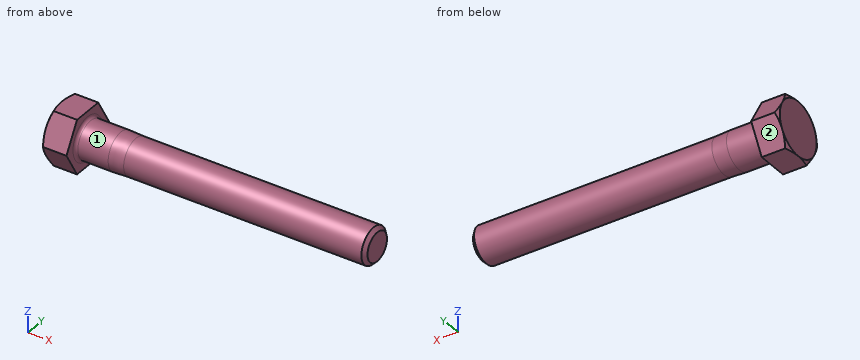
Autodesk Inventor part; units mm, degrees
ref_plane "Work Plane1" through (1.525, 0, 0) normal (0, 0, 1) x (1, 0, 0)
ref_plane "YZ Plane" through (0, 0, 0) normal (1, 0, 0) x (0, 1, 0)
ref_plane "XZ Plane" through (0, 0, 0) normal (0, 1, 0) x (-1, 0, 0)
sketch "Sketch1" plane through (0, 0, 0) normal (0, 0, 1) x (1, 0, 0)
  line L0 (0, 7.1374) -> (0, 4.9276)
  line L1 (12.7, 4.7625) -> (76.2, 4.7625)
  line L2 (76.2, 4.7625) -> (76.2, 0)
  line L3 (76.2, 0) -> (-0.0001, 0)
  line L4 (-15.2401, 0) -> (91.44, 0)
  line L5 (-0.0001, 0) -> (-0.0001, 7.1374)
  line L6 (-0.0001, 7.1374) -> (0, 7.1374)
  line L7 (12.7, 4.7625) -> (8.7311, 4.9276)
  line L8 (8.7311, 4.9276) -> (0, 4.9276)
  line L9 (0, -1.4275) -> (0, 8.5649)
  dimension "d0" = 76.2
  dimension "d1" = 63.5
revolve "Body" add sketch "Sketch1" angle 360 about axis through (76.2, 0, 0) along (-1, 0, 0)
sketch "Sketch2" plane through (-0.0001, 0, 0) normal (-1, 0, 0) x (0, 0, 1)
  line L0 (0, 8.2416) -> (7.1374, 4.1208)
  line L1 (7.1374, 4.1208) -> (7.1374, -4.1208)
  line L2 (7.1374, -4.1208) -> (0, -8.2416)
  line L3 (0, -8.2416) -> (-7.1374, -4.1208)
  line L4 (-7.1374, -4.1208) -> (-7.1374, 4.1208)
  line L5 (-7.1374, 4.1208) -> (0, 8.2416)
  point P0 (0, 0)
  point P1 (0, 0)
  dimension "d11" = 14.2748
extrude "Head" add sketch "Sketch2" along normal blind 6.8072
sketch "Sketch4" plane through (0, 0, 0) normal (0, 0, 1) x (1, 0, 0)
  line L0 (-6.8073, 7.1374) -> (-6.8073, 8.2416)
  line L1 (-6.8073, 8.2416) -> (-6.1698, 8.2416)
  line L2 (-6.1698, 8.2416) -> (-6.8073, 7.1374)
  line L3 (-8.1687, 0) -> (1.3613, 0)
  line L4 (-0.0001, 8.2416) -> (-6.8073, 8.2416)
  line L5 (-6.8073, 4.1208) -> (-6.8073, 8.2416)
  dimension "d5" = 30
  dimension "d19" = 14.2748
revolve "Chamfer1" cut sketch "Sketch4" angle 360 about axis through (-10, 0, 0) along (1, 0, 0)
thread "Thread"
chamfer "Chamfer2" distance 0.9739 distance2 0.9447 1 edges at (76.2, -4.7625, 0) measured on face at (76.2, -0.5629, 0.6211)
ref_plane "Work Plane1" through (1.525, 0, 0) normal (0, 0, 1) x (1, 0, 0)
fillet "Fillet2" radius 0.762 1 edges at (0, -4.9276, 0)
equation "\"d63\" = R"
equation "\"d11\" = SW"
equation "\"d3\" = KOH - SD"
equation "\"d15\" = GEL"
equation "\"d6\" = -0.5 * SPD + 0.5 * GD"
equation "\"d5\" = ANG1"
equation "\"d19\" = SW0"
equation "\"NLG\" = 190.5"
equation "\"GD\" = NND"
equation "\"BDM\" = 9.8552"
equation "\"KOH\" = 6.8072"
equation "\"GEL\" = 31.75"
equation "\"SW\" = 14.2748"
equation "\"SW0\" = SW"
equation "\"SPD\" = GD1"
equation "\"SD2\" = SW"
equation "\"SD\" = 0"
equation "\"ANG1\" = 30deg"
equation "\"GAL\" = 3.96875"
equation "\"GUL\" = 0.238 * GAL"
equation "\"R\" = 0.762"
equation "\"d62\" = -NLG - SD + GUL"
equation "\"GD1\" = 7.5773"
equation "\"THREADDIA\" = 9.525"
equation "\"TOA\" = 30deg"
equation "\"NND\" = 9.525"
equation "\"E0\" = 1.155 * SW"
properties part number "am-1055" material "Steel, Mild"
Input: part model. Units: mm. Frame: model coordinates. Face numbers are marked on the shaded views. A direction names the side the tool comes from. Round coordinates to 2 decimals unless told otherwise and drop trailing zeros. Loops run counter-clockwise (first coordinate to the right, second up) from the corner with the lowest first, then second, coordinate; pieces in that order, holes last. Notation, with made-up numbers: (-8, 84) -> (9, 84) arc R30 ccw to (9, 117) -> close; hole circle Ø5 at (74, -14). An arc over 180 degrees is marked (long way). Use one line per item in the form item = value. Start each with the question number.
Item 1: Material intervals for L1, parallel to X at y = -6, z = -3.5; L2, parallel to Z at x = 65, y = -0.75; L3, parallel to Z at x = 3, y = 2.75, sorted ascending. Write a range as from..to.
Item 2: Contact query for flat-ended pins moving along their axis: pin 1 Ø5 at (y, z) = (-6.5, -3) entering from +X; pin 2 Ø3 at (x, y) = (11, 3) entering from +Z; pin 3 Ø6 at (x, y) = (20, 5) entering from +Z. Output: stop coordinate, or through.
Item 3: Section query A-A on x = 63. Return the cut outline in (y, z) (1 decimal), then the cut area to 3 significant figures.
Item 4: Set-up query: the marked faces 1 and 2. Return all of +Z, -Z, +X, -X, +Y, -Y with unobstructed straight access to the full face (end or side cutting, diameter ignored); none if empty.
Ans:
q1.L1 = -6.81..0
q1.L2 = -4.7..4.7
q1.L3 = -4.09..4.09
q2.pin_1 = 75.36
q2.pin_2 = 4.6
q2.pin_3 = 4.32
q3.outline = circle Ø9.5 at (0, 0)
q3.area = 71.3 mm^2
q4.face_1 = +X
q4.face_2 = -Z, +X, -X, +Y
